Design review of the part built by this model. Coordinates are the model's own, in mm. Face numbers are marked on the shaded views. Coordinates: 2 decimals unless noted, no trailing zeros. Loops run counter-clockwise (first coordinate to the right, second up) from the corner with the lowest first, then second, coordinate; pieces in that order, holes last.
from build123d import *
from build123d.topology import SkipClean

# Parameters (mm, degrees)
EXTRUDE_3_DEPTH              = 1.5
EXTRUDE_3_2_DEPTH            = 1.5
SKETCH_2_R                   = 3.75
SKETCH_2_R_2                 = 2.5
EXTRUDE_5_DEPTH              = 3
EXTRUDE_START                = 2
SKETCH_3_R                   = 3.75
SKETCH_3_R_2                 = 2.5
EXTRUDE_6_DEPTH              = 2
ESQUISSE1_R                  = 0.587851578
ESQUISSE1_R_2                = 0.638983792
ENL_V_MAT_EXTRU_1_DEPTH      = 10
R_P_TITION_CIRCULAIRE1_COUNT = 2


with BuildPart() as part:
    # Sketch 1 → Extrude 3 (new body)
    with BuildSketch(Plane.XY):
        with BuildLine():
            ThreePointArc((-3.079299832, -2.140189839), (-3.57839869, -1.121411082), (-3.75, 0))
            ThreePointArc((-3.75, 0), (-3.57839869, 1.121411082), (-3.079299832, 2.140189839))
            Line((-3.079299832, 2.140189839), (-7.07082784, 1.998745461))
            ThreePointArc((-7.07082784, 1.998745461), (-9, 0), (-7.07082784, -1.998745461))
            Line((-7.07082784, -1.998745461), (-3.079299832, -2.140189839))
        make_face()
    extrude_3 = extrude(amount=EXTRUDE_3_DEPTH)



with BuildPart() as body_2:
    # Sketch 1 → Extrude 3 2 (new body)
    with BuildSketch(Plane.XY):
        with BuildLine():
            Line((3.079299832, 2.140189839), (1.172975936, 2.207742615))
            ThreePointArc((1.172975936, 2.207742615), (2.5, 0), (1.172975936, -2.207742615))
            Line((1.172975936, -2.207742615), (3.079299832, -2.140189839))
            ThreePointArc((3.079299832, -2.140189839), (3.75, 0), (3.079299832, 2.140189839))
        make_face()
    extrude_3_2 = extrude(amount=EXTRUDE_3_2_DEPTH)


with BuildPart() as body_3:
    # Sketch 2 → Extrude 5 (new body)
    with BuildSketch(Plane.XY.offset(1.5)):
        Circle(SKETCH_2_R)
        Circle(SKETCH_2_R_2, mode=Mode.SUBTRACT)
    extrude(amount=EXTRUDE_5_DEPTH)


with BuildPart() as part_1:
    with SkipClean():  # the faces are left unmerged after this step: merging them gives an invalid solid
        add(part.part)

        add(body_2.part)  # Extrude 6 merges body 2

        add(body_3.part)  # Extrude 6 merges body 3
        # Sketch 3 → Extrude 6 (add)
        with BuildSketch(Plane(origin=(0, 0, 1.5), x_dir=(-1, 0, 0), z_dir=(0, 0, -1)).offset(EXTRUDE_START)):
            Circle(SKETCH_3_R)
            Circle(SKETCH_3_R_2, mode=Mode.SUBTRACT)
        extrude(amount=-EXTRUDE_6_DEPTH)

    # Esquisse1 → Enl_v. mat.-Extru.1 (cut)
    with SkipClean():  # the faces are left unmerged after this step: merging them gives an invalid solid
        with BuildSketch(Plane.XY.offset(1.5)):
            with Locations((-4.5, 0)):
                Circle(ESQUISSE1_R)
            with Locations((-6.5, 0)):
                Circle(ESQUISSE1_R_2)
        enl_v_mat_extru_1 = extrude(amount=-ENL_V_MAT_EXTRU_1_DEPTH, mode=Mode.SUBTRACT)

    # R_p_tition circulaire1: Extrude 3, Extrude 3 2, Enl_v. mat.-Extru.1 ×2 about axis
    with SkipClean():  # the faces are left unmerged after this step: merging them gives an invalid solid
        r_p_tition_circulaire1_axis = Axis((0, 0, 0), (0, 0, 1))
        add([extrude_3.rotate(r_p_tition_circulaire1_axis, i * 360 / R_P_TITION_CIRCULAIRE1_COUNT) for i in range(1, R_P_TITION_CIRCULAIRE1_COUNT)])
        add([extrude_3_2.rotate(r_p_tition_circulaire1_axis, i * 360 / R_P_TITION_CIRCULAIRE1_COUNT) for i in range(1, R_P_TITION_CIRCULAIRE1_COUNT)])
        add([enl_v_mat_extru_1.rotate(r_p_tition_circulaire1_axis, i * 360 / R_P_TITION_CIRCULAIRE1_COUNT) for i in range(1, R_P_TITION_CIRCULAIRE1_COUNT)], mode=Mode.SUBTRACT)
    add(part_1.part.scale(1), mode=Mode.REPLACE)  # the faces are merged on a copy


solid = part_1.part
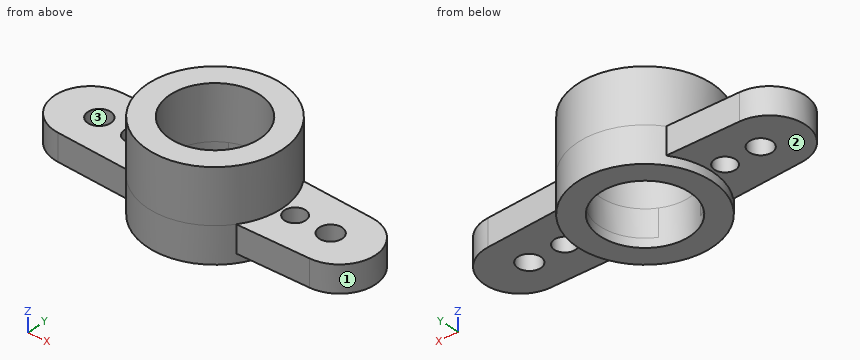
Q1. Take a section at C-C, the plane z = 3.65. Write out the cut boundary in (x, y), then the cut area to 3 significant figures.
Q2. Clearance check with flat-ended pins moving along their axes: pin 1 Ø1 at (y, z) = (1.5, 3) entering from -X; pin 2 Ø2 at (y, z) = (-2, 3) entering from +X; pin 3 Ø1.3 at (x, y) = (4.5, -0.5) entering from -Z. State where each tip first meets the part, or that it passes through.
Q3. Take a section at B-B, the plane z = 1.3. Write out the cut boundary in (x, y).
Q4. The part is to be moulded in two halves that separate along X. For the marked faces 1, 2 and 3, say which applies: pulls with the +X half, pulls with the -X half, needs draft (parallel to the pull), parting line crosses it, or undercut.
Q5. Take a section at D-D, the plane x = -4.5. Write out the cut boundary in (y, z), then the cut area to 3 significant figures.
Q6. For line 1 (Y direction, x = 0, z = 2.85); line 2 (X direction, y = 0.5, z = 1); line 3 (Y direction, x = -4.5, z = 1.05), list the stretches that pass through material, from the lowest coordinate up.
Q7. Take a section at A-A, the plane x = 0. Write out the cut boundary in (y, z), then the cut area to 3 significant figures.
Entries:
1. outline: circle Ø7.5 at (0, 0); hole circle Ø5 at (0, 0)
1. area: 24.5 mm2
2. pin 1: stops at x = -3.61
2. pin 2: stops at x = 3.61
2. pin 3: stops at z = 0
3. outline: (-7.07, -2) - (-3.08, -2.14) arc R3.75 ccw to (3.08, -2.14) - (7.07, -2) arc R2 ccw to (7.07, 2) - (3.08, 2.14) arc R3.75 ccw to (-3.08, 2.14) - (-7.07, 2) arc R2 ccw to start; hole circle Ø1.28 at (-6.5, 0); hole circle Ø1.18 at (-4.5, 0); hole circle Ø5 at (0, 0); hole circle Ø1.18 at (4.5, 0); hole circle Ø1.28 at (6.5, 0)
4. face 1: pulls with the +X half
4. face 2: needs draft
4. face 3: undercut
5. outline: (-2.09, 0) - (-0.59, 0) - (-0.59, 1.5) - (-2.09, 1.5) - close; (0.59, 0) - (2.09, 0) - (2.09, 1.5) - (0.59, 1.5) - close
5. area: 4.51 mm2
6. line 1: y = -3.75 to -2.5, 2.5 to 3.75
6. line 2: x = -8.94 to -6.9, -6.1 to -4.81, -4.19 to -2.45, 2.45 to 4.19, 4.81 to 6.1, 6.9 to 8.94
6. line 3: y = -2.09 to -0.59, 0.59 to 2.09
7. outline: (-3.75, -0.5) - (-2.5, -0.5) - (-2.5, 4.5) - (-3.75, 4.5) - close; (2.5, -0.5) - (3.75, -0.5) - (3.75, 4.5) - (2.5, 4.5) - close
7. area: 12.5 mm2
